Read the model definition and answer for the solid it produces. Units are mm, in the model's axes. A direction names the side the tool comes from. Coordinates: 2 decimals unless noted, no trailing zeros. Write each loop counter-clockwise with the first axis right and the second up, starting at its lowest first coordinate (ties: lowest second). Pieces come first, ordered by that corner, then holes. Notation, with made-up numbers: (-32, 18) - (-22, 18) arc R23 ccw to (-22, 45) - close; hole circle Ø3 at (-36, 28.25). An arc over 180 degrees is marked (long way). Use a Markdown table: item, result.
Autodesk Inventor part; units mm, degrees
ref_plane "YZ Plane" through (0, 0, 0) normal (1, 0, 0) x (0, 1, 0)
ref_plane "XZ Plane" through (0, 0, 0) normal (0, 1, 0) x (-1, 0, 0)
ref_plane "XY Plane" through (0, 0, 0) normal (0, 0, 1) x (1, 0, 0)
sketch "Sketch1" plane through (0, 0, 0) normal (0, 0, 1) x (1, 0, 0)
  line L0 (-11.5, -17.5) -> (11.5, -17.5)
  line L1 (11.5, -17.5) -> (11.5, 17.5)
  line L2 (11.5, 17.5) -> (-11.5, 17.5)
  line L3 (-11.5, 17.5) -> (-11.5, -17.5)
  line L4 (-11.5, -17.5) -> (11.5, 17.5) construction
  line L5 (11.5, -17.5) -> (-11.5, 17.5) construction
  line L6 (-11.5, 4.5) -> (-16, 4.5)
  line L7 (-20.5, 0) -> (-20.5, 0)
  line L8 (-16, -4.5) -> (-11.5, -4.5)
  line L9 (11.5, 4.5) -> (16, 4.5)
  line L10 (20.5, 0) -> (20.5, 0)
  line L11 (16, -4.5) -> (11.5, -4.5)
  arc A0 (16, -4.5) -> (20.5, 0) centre (16, 0) ccw
  arc A1 (20.5, 0) -> (16, 4.5) centre (16, 0) ccw
  arc A2 (-20.5, 0) -> (-16, -4.5) centre (-16, 0) ccw
  arc A3 (-16, 4.5) -> (-20.5, 0) centre (-16, 0) ccw
  point P0 (0, 0)
  point P1 (-20.5, 0)
  point P2 (-11.5, 0)
  point P3 (20.5, 0)
  point P4 (11.5, 0)
  point P5 (13.75, -4.5)
  point P6 (0, -17.5)
  point P7 (20.5, 0)
  dimension "d0" = 35
  dimension "d1" = 23
  dimension "d2" = 4.5
  dimension "d3" = 9
  dimension "d4" = 4.5
  dimension "d5" = 9
  dimension "d6" = 32
  dimension "d7" = 16
extrude "Extrusion1" add sketch "Sketch1" along normal mid plane 15
sketch "Sketch2" plane through (0, 0, 7.5) normal (0, 0, 1) x (1, 0, 0)
  arc A0 (-16, 4.5) -> (-16, -4.5) centre (-16, 0) ccw
  arc A1 (16, -4.5) -> (16, 4.5) centre (16, 0) ccw
  point P0 (0, 0)
  point P1 (-16, 0)
  point P2 (16, 0)
hole "Hole1" at (-16, 0, 7.5) at (16, 0, 7.5) direction (0, 0, -1) diameter 4.917 depth 15
sketch "Sketch4" plane through (-11.5, 17.5, 7.5) normal (0, 1, 0) x (1, 0, 0)
  point P0 (11.5, 7.5)
  point P1 (11.5, 7.5)
hole "Hole2" at (0, 17.5, 0) direction (0, -1, 0) diameter 5.9175 end through all
sketch "Sketch3" plane through (0, 0, 7.5) normal (0, 0, 1) x (1, 0, 0)
  line L0 (-5, -15) -> (5, -15)
  line L1 (5, -15) -> (5, 15)
  line L2 (5, 15) -> (-5, 15)
  line L3 (-5, 15) -> (-5, -15)
  line L4 (-5, -15) -> (5, 15) construction
  line L5 (5, -15) -> (-5, 15) construction
  point P0 (0, 0)
  dimension "d17" = 10
  dimension "d18" = 30
extrude "Extrusion2" cut sketch "Sketch3" against normal blind 10
sketch "Sketch6" plane through (0, 0, 7.5) normal (0, 0, 1) x (1, 0, 0)
  line L0 (-11.5, -17.5) -> (11.5, -17.5)
  point P0 (0, 0)
  point P1 (-9, -13)
  point P2 (-9, -5)
  point P3 (9, -5)
  point P4 (9, -13)
  dimension "d31" = 8
  dimension "d42" = 5
  dimension "d43" = 18
  dimension "d44" = 9
hole "Hole3" at (-9, -13, 7.5) at (-9, -5, 7.5) at (9, -5, 7.5) at (9, -13, 7.5) direction (0, 0, -1) diameter 2.5 depth 15
mirror "Mirror1" about plane through (0, 0, 0) normal (0, 1, 0) of "Hole3"
fillet "Fillet1" radius 2.5 6 edges at (11.5, 17.5, 3.75) (11.5, 17.5, -3.75) (-11.5, 17.5, 3.75) (-11.5, 17.5, -3.75) (-11.5, -17.5, 0) (11.5, -17.5, 0)
equation "\"d5\" = d3"
properties part number "15"
(1) A cutting plane is placed at A-A, the plane y = -13. Write down the section's boundary in (x, z).
Report:
| item | result |
|---|---|
| outline | (-11.5, -7.5) - (-10.25, -7.5) - (-10.25, 7.5) - (-11.5, 7.5) - close; (-7.75, -7.5) - (7.75, -7.5) - (7.75, 7.5) - (5, 7.5) - (5, -2.5) - (1.58, -2.5) arc R2.96 cw to (-1.58, -2.5) - (-5, -2.5) - (-5, 7.5) - (-7.75, 7.5) - close; (10.25, -7.5) - (11.5, -7.5) - (11.5, 7.5) - (10.25, 7.5) - close |
(2) For faces 4 (the flat face through (11.5, 10, 0)), 5 (the flat face through (-14, -4.5, 0)), 6 (the flat face through (11.5, -10, 0)), 7 (the flat face through (-5, 0, 3)), determine the directions among +Z, -Z, +X, -X, +Y, -Y from which every point of the face is accessible in a straight line to the end or side of a thin tool.
Report:
| item | result |
|---|---|
| face 4 | +Z, -Z, +X, +Y |
| face 5 | +Z, -Z, -X, -Y |
| face 6 | +Z, -Z, +X, -Y |
| face 7 | +Z |
(3) Each of these flat-tipped pins is pushed along its axis until it touches: P1, Ø1, axis at x = 3, y = 6.5, coming from the +Z side; P2, Ø3, axis at y = 12.5, z = 2.5, coming from the +X side; P3, Ø4, axis at y = -9.5, z = 1, coming from the -X side; P4, Ø5.5, axis at x = 16, y = 0, coming from the -Z side. Where does it stop, or does it pass through?
Report:
| item | result |
|---|---|
| P1 | stops at z = -2.5 |
| P2 | stops at x = 11.5 |
| P3 | stops at x = -11.5 |
| P4 | stops at z = -7.5 |
(4) A cutting plane is placed at C-C, the plane z = 4.5. Count the separate pieces of the cut face and the enclosed holes in it, and give its area (3 significant figures).
Report:
| item | result |
|---|---|
| separate pieces | 1 |
| enclosed holes | 11 |
| area | 567 mm² |
(5) The mould has two halves that part along Y. Classify faces 1 (the cylindrical face through (-10.748, 16.787, 0.105)), 2 (the cylindrical face through (-10.24, -12.84, -0.11)), 3 (the cylindrical face through (10.748, -16.787, 0.105)): pulls with the +Y half, pulls with the -Y half, needs draft (parallel to the pull), parting line crosses it, or undercut.
Report:
| item | result |
|---|---|
| face 1 | pulls with the +Y half |
| face 2 | undercut |
| face 3 | pulls with the -Y half |
(6) A cutting plane is placed at B-B, the plane x = 0. Write down the section's boundary in (y, z).
Report:
| item | result |
|---|---|
| outline | (-17.5, -7.5) - (17.5, -7.5) - (17.5, -2.96) - (-17.5, -2.96) - close; (-17.5, 2.96) - (-15, 2.96) - (-15, 7.5) - (-17.5, 7.5) - close; (15, 2.96) - (17.5, 2.96) - (17.5, 7.5) - (15, 7.5) - close |
(7) Straight lines are drawn through the part: L1, parallel to X at y = 0, z = 1; L2, parallel to Y at x = 9, z = 4; L3, parallel to X at y = 5, z = 3.5. For each, find the intervals that lie inside material, in ascending order.
Report:
| item | result |
|---|---|
| L1 | x = -20.5 to -18.46, -13.54 to -5, 5 to 13.54, 18.46 to 20.5 |
| L2 | y = -17.5 to -14.25, -11.75 to -6.25, -3.75 to 3.75, 6.25 to 11.75, 14.25 to 17.5 |
| L3 | x = -11.5 to -10.25, -7.75 to -5, 5 to 7.75, 10.25 to 11.5 |
